Can you work these out from the drawing? Everything is in mm from the part's minimum corner. Round coordinates to 2 decimals unless told otherwise and drop trailing zeros. Order: outer loops, then holes, each group sorted by start corner. A loop starts at its lowest first (then second) coordinate and runs counter-clockwise, first axis right, second up. Notation, with made-up numbers: (20.25, 68) - (79.25, 68) arc R14 ccw to (79.25, 89) - close; hole circle Ø2 at (18, 78.5). An arc over 180 degrees is marked (long way). Write item = value, one per line.
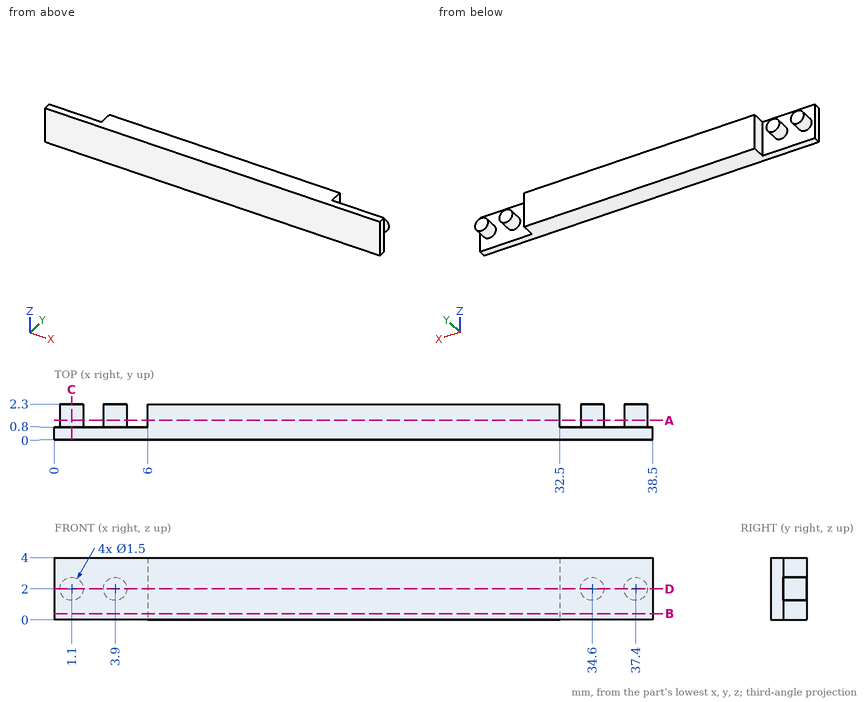
(1) If we section it at D-D (z = 2): Write out the boundary of the cut face in (x, y), plus the area to 4 significant figures.
Computed:
outline = (0, 0) - (38.5, 0) - (38.5, 0.8) - (38.15, 0.8) - (38.15, 2.3) - (36.65, 2.3) - (36.65, 0.8) - (35.35, 0.8) - (35.35, 2.3) - (33.85, 2.3) - (33.85, 0.8) - (32.5, 0.8) - (32.5, 2.3) - (6, 2.3) - (6, 0.8) - (4.65, 0.8) - (4.65, 2.3) - (3.15, 2.3) - (3.15, 0.8) - (1.85, 0.8) - (1.85, 2.3) - (0.35, 2.3) - (0.35, 0.8) - (0, 0.8) - close
area = 79.55 mm^2
(2) If we section it at A-A (y = 1.25): Write out the boundary of the cut face in (x, z), plus the area to 3 significant figures.
Computed:
outline = circle Ø1.5 at (1.1, 2); circle Ø1.5 at (3.9, 2); (6, 0) - (32.5, 0) - (32.5, 4) - (6, 4) - close; circle Ø1.5 at (34.6, 2); circle Ø1.5 at (37.4, 2)
area = 113 mm^2
(3) If we section it at C-C (x = 1.1): Write out the boundary of the cut face in (y, z).
Computed:
outline = (0, 0) - (0.8, 0) - (0.8, 1.25) - (2.3, 1.25) - (2.3, 2.75) - (0.8, 2.75) - (0.8, 4) - (0, 4) - close
(4) If I drill on line 1 (X direction, y = 0.85, z = 2.05); line 2 (X direction, y = 2.05, z = 1.6); line 3 (Y direction, x = 36, z = 0.65), over which ranges is the centre line in solid material (lowest first)? Write a range as from..to.
Computed:
line_1 = 0.35..1.85, 3.15..4.65, 6..32.5, 33.85..35.35, 36.65..38.15
line_2 = 0.47..1.73, 3.27..4.53, 6..32.5, 33.97..35.23, 36.77..38.03
line_3 = 0..0.8
(5) Will this pin go through, and if not, where does the flat tip stop? P1, Ø1.2, axis at x = 35.5, z = 2, coming from the +Y side.
Computed:
P1 = 2.3
(6) If we section it at B-B (z = 0.4): Write out the boundary of the cut face in (x, y), plus the area to 4 significant figures.
Computed:
outline = (0, 0) - (38.5, 0) - (38.5, 0.8) - (32.5, 0.8) - (32.5, 2.3) - (6, 2.3) - (6, 0.8) - (0, 0.8) - close
area = 70.55 mm^2
